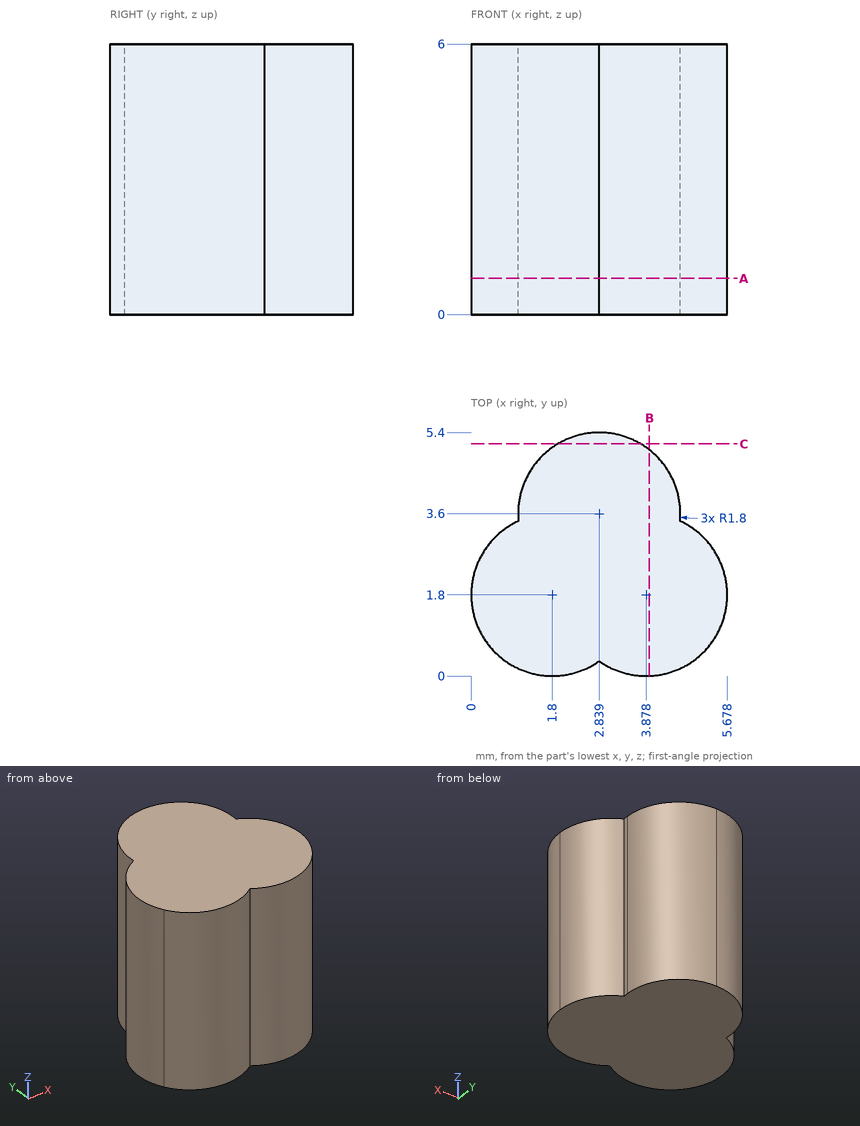
Here's the drawing with two shaded views (mm, measured from the low corner). I have some questions. Coordinates: 2 decimals unless noted, no trailing zeros. Loops run counter-clockwise (first coordinate to the right, second up) from the corner with the lowest first, then second, coordinate; pieces in that order, holes last. Notation, with made-up numbers: M 41,39.25 L 94,39.25 A9 ccw 94,53.25 Z; hole C 9.25,70.5 d5. An arc over 180 degrees is marked long. Put each result on its own line as item: value. Start each with the question number.
(1) Imagine slicing it at A-A on z = 0.8. List the corners of the cut face in (x, y) for me (1 decimal), and give its area (3 significant figures).
(2) I need wall thicknesses on probe 1 along Y at (x, z) = (3.15, 3.7) (1 decimal); probe 2 along Y at (x, z) = (4.75, 5.45) (1 decimal); probe 3 along X at (y, z) = (3.85, 1.95). Which ranges of each line are inside material? Lowest first, please.
(3) Imagine slicing it at C-C on y = 5.15. List the corners of the cut face in (x, z) for me (1 decimal).
(4) Imagine slicing it at B-B on x = 3.95. List the corners of the cut face in (y, z) for me.
Worked answers:
1. outline: M 1,3.4 A1.8 ccw long 2.8,0.3 A1.8 ccw long 4.6,3.4 A1.8 ccw long Z
1. area: 22.6 mm2
2. probe 1: y = 0.2 to 5.4
2. probe 2: y = 0.2 to 3.4
2. probe 3: x = 1.06 to 4.62
3. outline: M 1.9,0 L 3.8,0 L 3.8,6 L 1.9,6 Z
4. outline: M 0,0 L 5.02,0 L 5.02,6 L 0,6 Z
